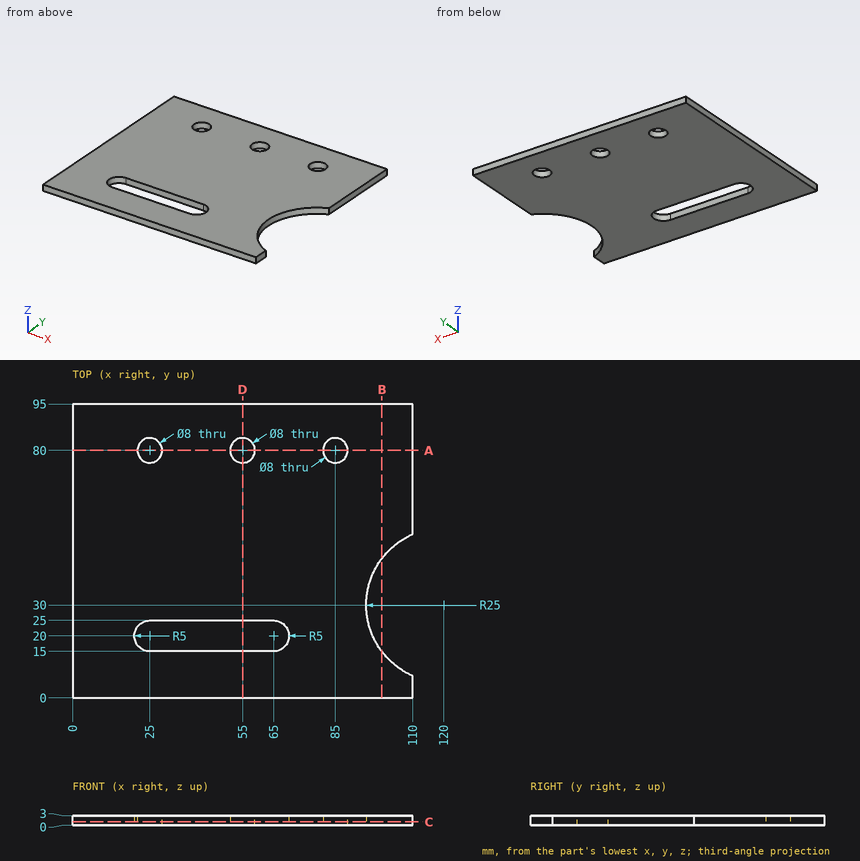
Input: dimensioned drawing with shaded views. Units: mm. Origin: part minimum x, y, z. Give positions to 0.01 mm unless a question says otherwise; leave off trailing zeros. Write each loop counter-clockwise with the first axis right and the second up, starting at its lowest first coordinate (ties: lowest second). Pieces come first, ordered by that corner, then holes.
1. Section query B-B, the plane x = 100. Return loops of the section in (y, z), then the cut area to 3 significant figures.
2. Section query D-D, the plane x = 55. Return loops of the section in (y, z).
3. Pin query (flat end, axial travel): P1, Ø6, axis at x = 38, y = 43, coming from the -Z side; P2, Ø5, axis at x = 25, y = 80, coming from the -Z side. Return the tip coordinate at first contact, or that it passes through.
4. Line query: probe 1 along Y at (x, z) = (25, 1.7); probe 2 along Y at (x, z) = (65.5, 2.4); probe 3 along Y at (x, z) = (98.5, 1.35). Output: solid intervals per line, ascending.
5. Section query C-C, the plane z = 1. Return loops of the section in (x, y), then the cut area to 3 significant figures.
6. Section query A-A, the plane y = 80. Return loops of the section in (x, z).
Computed:
1. outline: (0, 0) - (15, 0) - (15, 3) - (0, 3) - close; (45, 0) - (95, 0) - (95, 3) - (45, 3) - close
1. area: 195 mm2
2. outline: (0, 0) - (15, 0) - (15, 3) - (0, 3) - close; (25, 0) - (76, 0) - (76, 3) - (25, 3) - close; (84, 0) - (95, 0) - (95, 3) - (84, 3) - close
3. P1: stops at z = 0
3. P2: passes through
4. probe 1: y = 0 to 15, 25 to 76, 84 to 95
4. probe 2: y = 0 to 15.03, 24.97 to 95
4. probe 3: y = 0 to 17.24, 42.76 to 95
5. outline: (0, 0) - (110, 0) - (110, 7.09) arc R25 cw to (110, 52.91) - (110, 95) - (0, 95) - close; hole circle Ø8 at (25, 80); hole (25, 15) - (65, 15) arc R5 ccw to (65, 25) - (25, 25) arc R5 ccw to start; hole circle Ø8 at (55, 80); hole circle Ø8 at (85, 80)
5. area: 9,330 mm2
6. outline: (0, 0) - (21, 0) - (21, 3) - (0, 3) - close; (29, 0) - (51, 0) - (51, 3) - (29, 3) - close; (59, 0) - (81, 0) - (81, 3) - (59, 3) - close; (89, 0) - (110, 0) - (110, 3) - (89, 3) - close
